The figure shows three views and two pictorial views of one solid part (mm, origin at its lowest corner). Answer the questions. A direction names the side the tool comes from. Coordinates: 2 decimals unless noted, no trailing zeros. Order: outer loops, then holes, each group sorted by start corner. A loop starts at its lowest first (then second) coordinate and runs counter-clockwise, first axis right, second up. Notation, with made-up numbers: (83.5, 9) - (108.5, 9) arc R13 ccw to (108.5, 28) - close; hole circle Ø5 at (24.5, -22). An arc over 180 degrees is marked (long way). Use one line per item in the form item = value.
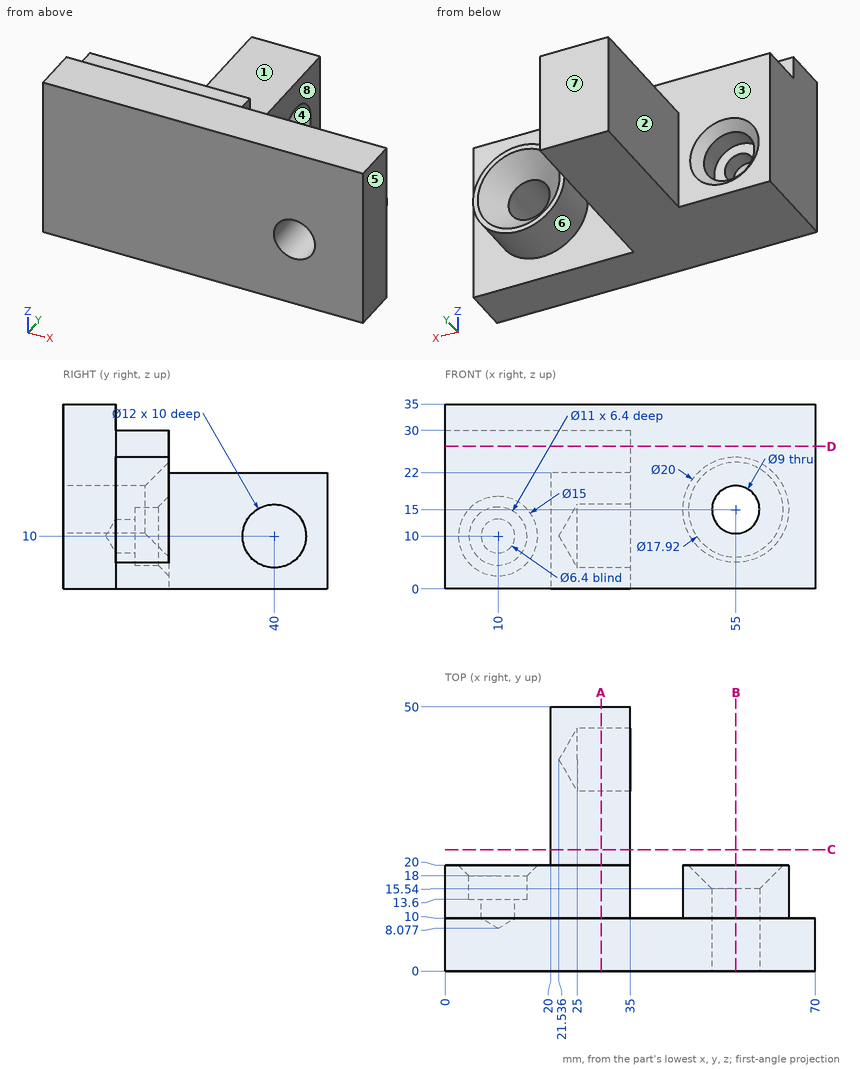
(1) Given pin 1 Ø6 at (y, z) = (11, 17.5) entering from +X; pin 2 Ø1 at (y, z) = (15, 17) entering from +X; pin 3 Ø4.5 at (x, y) = (31, 33.5) entering from +Z; pin 4 Ø11.5 at (x, z) = (55, 15) entering from +Y, each flat-ended and moving along its own axis, determine where each tip first touches the part or whether it passes through.
Answer list:
pin_1 = 70
pin_2 = 64.89
pin_3 = 22
pin_4 = 16.79
(2) Section D-D, the plane z = 27 is taken. Write down the section's boundary in (x, y).
Answer list:
outline = (0, 0) - (70, 0) - (70, 10) - (35, 10) - (35, 20) - (0, 20) - close
(3) Section A-A, the plane x = 29.5 is taken. Write down the section's boundary in (y, z), then the cut area to 3 significant figures.
Answer list:
outline = (0, 0) - (50, 0) - (50, 22) - (20, 22) - (20, 30) - (10, 30) - (10, 35) - (0, 35) - close; hole circle Ø12 at (40, 10)
area = 1,200 mm2
(4) Which of the six approach directions +Z, -Z, +X, -X, +Y, -Y give full straight-line access (tool end or side, diameter ignored) to the marked faces 1, 2, 3 and 4?
Answer list:
face_1 = +Z, +X, -X, +Y
face_2 = +Z, -Z, -X, +Y
face_3 = +Z, -X, +Y
face_4 = +X
(5) Section B-B, the plane x = 55 is taken. Write down the section's boundary in (y, z).
Answer list:
outline = (0, 0) - (10, 0) - (10, 5) - (20, 5) - (20, 6.04) - (15.54, 10.5) - (0, 10.5) - close; (0, 19.5) - (15.54, 19.5) - (20, 23.96) - (20, 25) - (10, 25) - (10, 35) - (0, 35) - close
(6) Straight lines are drawn through the part: L1, parallel to X at y = 5.5, z = 15; L2, parallel to X at y = 18.5, z = 12; L3, parallel to Z at x = 10, y = 12. For each, find the intervals that lie inside material, in ascending order.
Answer list:
L1 = 0 to 50.5, 59.5 to 70
L2 = 0 to 4.34, 15.66 to 35, 45.46 to 48.17, 61.83 to 64.54
L3 = 0 to 6.8, 13.2 to 30
(7) Section C-C, the plane y = 23 is taken. Write down the section's boundary in (x, z).
Answer list:
outline = (20, 0) - (35, 0) - (35, 22) - (20, 22) - close
(8) The mould has two halves that part along X. Classify the marked faces 5, 6, 7 and 8: +X half, -X half, draft (parallel to the pull), parting line (faces both ways), or undercut.
Answer list:
face_5 = +X half
face_6 = undercut
face_7 = draft
face_8 = undercut
